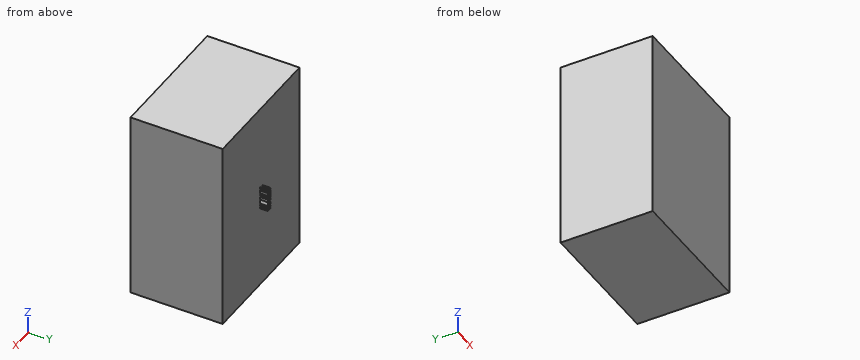
Autodesk Inventor part; units mm, degrees
ref_plane "YZ Plane" through (0, 0, 0) normal (1, 0, 0) x (0, 1, 0)
ref_plane "XZ Plane" through (0, 0, 0) normal (0, 1, 0) x (-1, 0, 0)
ref_plane "XY Plane" through (0, 0, 0) normal (0, 0, 1) x (1, 0, 0)
sketch "Boceto1" plane through (0, 0, 0) normal (0, 1, 0) x (-1, 0, 0)
  line L0 (42.5, 60) -> (-42.5, 60)
  line L1 (-42.5, 60) -> (-42.5, -60)
  line L2 (-42.5, -60) -> (42.5, -60)
  line L3 (42.5, -60) -> (42.5, 60)
  line L4 (42.5, 60) -> (-42.5, -60) construction
  line L5 (-42.5, 60) -> (42.5, -60) construction
  point P0 (0, 0)
  dimension "d0" = 85
  dimension "d1" = 120
extrude "Extrusión1" add sketch "Boceto1" along normal blind 58
sketch "Boceto2" plane through (0, 58, 0) normal (0, 1, 0) x (1, 0, 0)
  line L0 (-1.6968, -6.642) -> (-1.6968, 31.3478) construction
  line L1 (-1.6968, 31.3478) -> (74.717, 31.3478) construction
  line L2 (74.717, 31.3478) -> (74.717, -6.642) construction
  line L3 (74.717, -6.642) -> (-1.6968, -6.642) construction
  spline S0 degree 2 poles (0.6226, -5.1847) (1.0227, -5.1847) (1.4574, -5.6738) (1.4574, -6.0862) knots 0 0 0 1 2 2 2
  spline S1 degree 2 poles (1.4574, -6.0862) (1.4574, -6.185) (1.4229, -6.5136) (1.3982, -6.6247) knots 0 0 0 1 2 2 2
  line L4 (1.3982, -6.6247) -> (1.0079, -6.6247)
  line L5 (1.0079, -6.6247) -> (1.0079, -6.6025)
  spline S2 degree 2 poles (1.0079, -6.6025) (1.0375, -6.5185) (1.1067, -6.269) (1.1067, -6.1406) knots 0 0 0 1 2 2 2
  spline S3 degree 2 poles (1.1067, -6.1406) (1.1067, -5.9529) (1.0202, -5.7281) (0.9412, -5.6762) knots 0 0 0 1 2 2 2
  spline S4 degree 2 poles (0.9412, -5.6762) (0.8597, -5.6194) (0.6226, -5.5898) (0.467, -5.5898) knots 0 0 0 1 2 2 2
  line L6 (0.467, -5.5898) -> (-1.309, -5.5898)
  line L7 (-1.309, -5.5898) -> (-1.309, -6.2344)
  line L8 (-1.309, -6.2344) -> (-1.6326, -6.2344)
  line L9 (-1.6326, -6.2344) -> (-1.6326, -5.1847)
  line L10 (-1.6326, -5.1847) -> (0.6226, -5.1847)
  line L11 (1.4154, -4.5869) -> (-1.6326, -4.5869)
  line L12 (-1.6326, -4.5869) -> (-1.6326, -2.6801)
  line L13 (-1.6326, -2.6801) -> (-1.2719, -2.6801)
  line L14 (-1.2719, -2.6801) -> (-1.2719, -4.1819)
  line L15 (-1.2719, -4.1819) -> (-0.4371, -4.1819)
  line L16 (-0.4371, -4.1819) -> (-0.4371, -2.7814)
  line L17 (-0.4371, -2.7814) -> (-0.0764, -2.7814)
  line L18 (-0.0764, -2.7814) -> (-0.0764, -4.1819)
  line L19 (-0.0764, -4.1819) -> (1.0548, -4.1819)
  line L20 (1.0548, -4.1819) -> (1.0548, -2.6801)
  line L21 (1.0548, -2.6801) -> (1.4154, -2.6801)
  line L22 (1.4154, -2.6801) -> (1.4154, -4.5869)
  line L23 (1.4154, -1.5241) -> (-1.2719, -1.5241)
  line L24 (-1.2719, -1.5241) -> (-1.2719, -2.5467)
  line L25 (-1.2719, -2.5467) -> (-1.6326, -2.5467)
  line L26 (-1.6326, -2.5467) -> (-1.6326, -0.0965)
  line L27 (-1.6326, -0.0965) -> (-1.2719, -0.0965)
  line L28 (-1.2719, -0.0965) -> (-1.2719, -1.119)
  line L29 (-1.2719, -1.119) -> (1.4154, -1.119)
  line L30 (1.4154, -1.119) -> (1.4154, -1.5241)
  spline S5 degree 2 poles (1.4698, 1.062) (1.4698, 0.731) (1.3315, 0.2666) (1.2327, 0.0616) knots 0 0 0 1 2 2 2
  line L31 (1.2327, 0.0616) -> (0.7238, 0.0616)
  line L32 (0.7238, 0.0616) -> (0.7238, 0.0913)
  spline S6 degree 2 poles (0.7238, 0.0913) (0.9116, 0.2913) (1.119, 0.7977) (1.119, 1.0323) knots 0 0 0 1 2 2 2
  spline S7 degree 2 poles (1.119, 1.0323) (1.119, 1.3683) (0.8399, 1.7116) (0.6102, 1.7116) knots 0 0 0 1 2 2 2
  spline S8 degree 2 poles (0.6102, 1.7116) (0.4274, 1.7116) (0.2002, 1.5313) (0.1434, 1.3361) knots 0 0 0 1 2 2 2
  spline S9 degree 2 poles (0.1434, 1.3361) (0.1039, 1.1954) (0.0495, 0.9607) (0.0051, 0.7853) knots 0 0 0 1 2 2 2
  spline S10 degree 2 poles (0.0051, 0.7853) (-0.0369, 0.6273) (-0.1629, 0.3778) (-0.2642, 0.2815) knots 0 0 0 1 2 2 2
  spline S11 degree 2 poles (-0.2642, 0.2815) (-0.3654, 0.1876) (-0.6371, 0.0839) (-0.815, 0.0839) knots 0 0 0 1 2 2 2
  spline S12 degree 2 poles (-0.815, 0.0839) (-1.1855, 0.0839) (-1.6869, 0.6618) (-1.6869, 1.1089) knots 0 0 0 1 2 2 2
  spline S13 degree 2 poles (-1.6869, 1.1089) (-1.6869, 1.3658) (-1.5856, 1.8203) (-1.4893, 2.0154) knots 0 0 0 1 2 2 2
  line L33 (-1.4893, 2.0154) -> (-1.0052, 2.0154)
  line L34 (-1.0052, 2.0154) -> (-1.0052, 1.9858)
  spline S14 degree 2 poles (-1.0052, 1.9858) (-1.1386, 1.84) (-1.3362, 1.3856) (-1.3362, 1.1361) knots 0 0 0 1 2 2 2
  spline S15 degree 2 poles (-1.3362, 1.1361) (-1.3362, 0.8545) (-1.0719, 0.5062) (-0.857, 0.5062) knots 0 0 0 1 2 2 2
  spline S16 degree 2 poles (-0.857, 0.5062) (-0.6643, 0.5062) (-0.4346, 0.7112) (-0.3827, 0.9039) knots 0 0 0 1 2 2 2
  spline S17 degree 2 poles (-0.3827, 0.9039) (-0.3481, 1.0323) (-0.2592, 1.4053) (-0.2222, 1.5288) knots 0 0 0 1 2 2 2
  spline S18 degree 2 poles (-0.2222, 1.5288) (-0.1258, 1.8425) (0.2619, 2.134) (0.546, 2.134) knots 0 0 0 1 2 2 2
  spline S19 degree 2 poles (0.546, 2.134) (0.7263, 2.134) (1.0721, 1.9882) (1.1931, 1.8573) knots 0 0 0 1 2 2 2
  spline S20 degree 2 poles (1.1931, 1.8573) (1.3265, 1.7116) (1.4698, 1.3411) (1.4698, 1.062) knots 0 0 0 1 2 2 2
  spline S21 degree 2 poles (-1.2843, 4.7028) (-1.0817, 4.8757) (-0.4889, 5.0683) (-0.1086, 5.0683) knots 0 0 0 1 2 2 2
  spline S22 degree 2 poles (-0.1086, 5.0683) (0.2619, 5.0683) (0.8622, 4.8806) (1.0647, 4.7028) knots 0 0 0 1 2 2 2
  spline S23 degree 2 poles (1.0647, 4.7028) (1.2771, 4.5151) (1.4797, 4.0186) (1.4797, 3.7197) knots 0 0 0 1 2 2 2
  spline S24 degree 2 poles (1.4797, 3.7197) (1.4797, 3.411) (1.2697, 2.917) (1.0647, 2.7366) knots 0 0 0 1 2 2 2
  spline S25 degree 2 poles (1.0647, 2.7366) (0.8622, 2.5613) (0.2669, 2.3736) (-0.1086, 2.3736) knots 0 0 0 1 2 2 2
  spline S26 degree 2 poles (-0.1086, 2.3736) (-0.4914, 2.3736) (-1.0743, 2.5637) (-1.2843, 2.7391) knots 0 0 0 1 2 2 2
  spline S27 degree 2 poles (-1.2843, 2.7391) (-1.4868, 2.917) (-1.6968, 3.4134) (-1.6968, 3.7197) knots 0 0 0 1 2 2 2
  spline S28 degree 2 poles (-1.6968, 3.7197) (-1.6968, 4.0309) (-1.4794, 4.5299) (-1.2843, 4.7028) knots 0 0 0 1 2 2 2
  spline S29 degree 2 poles (-0.1086, 4.646) (-0.4099, 4.646) (-0.8767, 4.5151) (-1.0299, 4.3965) knots 0 0 0 1 2 2 2
  spline S30 degree 2 poles (-1.0299, 4.3965) (-1.188, 4.2755) (-1.346, 3.9346) (-1.346, 3.7222) knots 0 0 0 1 2 2 2
  spline S31 degree 2 poles (-1.346, 3.7222) (-1.346, 3.5024) (-1.1929, 3.1714) (-1.0299, 3.0454) knots 0 0 0 1 2 2 2
  spline S32 degree 2 poles (-1.0299, 3.0454) (-0.8743, 2.9244) (-0.405, 2.7959) (-0.1086, 2.7959) knots 0 0 0 1 2 2 2
  spline S33 degree 2 poles (-0.1086, 2.7959) (0.4917, 2.7959) (1.1289, 3.2998) (1.1289, 3.7222) knots 0 0 0 1 2 2 2
  spline S34 degree 2 poles (1.1289, 3.7222) (1.1289, 4.1446) (0.4917, 4.646) (-0.1086, 4.646) knots 0 0 0 1 2 2 2
  line L35 (1.4154, 7.694) -> (1.4154, 7.2395)
  line L36 (1.4154, 7.2395) -> (-1.2127, 5.8909)
  line L37 (-1.2127, 5.8909) -> (1.4154, 5.8909)
  line L38 (1.4154, 5.8909) -> (1.4154, 5.5129)
  line L39 (1.4154, 5.5129) -> (-1.6326, 5.5129)
  line L40 (-1.6326, 5.5129) -> (-1.6326, 6.0885)
  line L41 (-1.6326, 6.0885) -> (0.7807, 7.3161)
  line L42 (0.7807, 7.3161) -> (-1.6326, 7.3161)
  line L43 (-1.6326, 7.3161) -> (-1.6326, 7.694)
  line L44 (-1.6326, 7.694) -> (1.4154, 7.694)
  point P0 (0, 0)
extrude "Extrusión2" add sketch "Boceto2" along normal blind 5
properties part number "jetson"
Can you work these out from the model? Positions are in its coordinate system, mm. Round coordinates to 2 decimals unless told otherwise and drop trailing zeros. Loops run counter-clockwise (first coordinate to the right, second up) from the corner with the lowest first, then second, coordinate; pieces in that order, holes last.
Item 1: Please list where this line runs through material, in increasing order: L1, parallel to Y at x = -32.5, z = -5.
Item 2: Will these pins go through, and if not, where does the flat tip stop? pin 1 Ø1.5 at (x, y) = (-1, 60) entering from +Z; pin 2 Ø0.8 at (y, z) = (60.5, 5.5) entering from -X; pin 3 Ø1 at (y, z) = (61, 3.5) entering from +X.
Item 3: Suppose I cut it at B-B, the plane z = 17. Write out the boundary of the cut face in (x, y), then the cut area to 3 significant figures.
Item 4: Suppose I cut it at A-A, the plane x = 19.5. Write out the boundary of the cut face in (y, z).
Reported:
1. L1: y = 0 to 58
2. pin 1: stops at z = 6.23
2. pin 2: stops at x = -1.63
2. pin 3: stops at x = 1.42
3. outline: (-42.5, 0) - (42.5, 0) - (42.5, 58) - (-42.5, 58) - close
3. area: 4,930 mm2
4. outline: (0, -60) - (58, -60) - (58, 60) - (0, 60) - close
